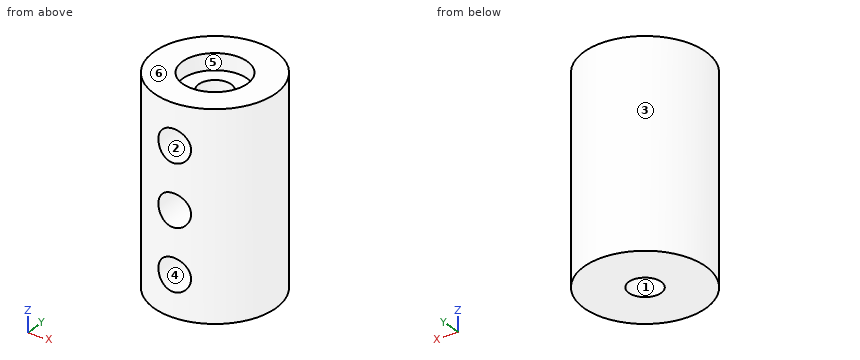
from build123d import *

# Parameters (mm, degrees)
F0_R     = 7.5
F0_R_2   = 2
F1_DEPTH = 12.5
F2_R     = 2
F3_DEPTH = 25
F4_R     = 4
F5_DEPTH = 2


with BuildPart() as f1:
    # F0 (on Top) → F1 (new body, symmetric)
    with BuildSketch(Plane.XY):
        Circle(F0_R)
        Circle(F0_R_2, mode=Mode.SUBTRACT)
    extrude(amount=F1_DEPTH, both=True)

    # F2 (on Front) → F3 (cut)
    with BuildSketch(Plane.XZ):
        with Locations((0, 7.5)):
            Circle(F2_R)
        with Locations((0, -7.5)):
            Circle(F2_R)
        Circle(F2_R)
    extrude(amount=F3_DEPTH, mode=Mode.SUBTRACT)

    # F4 (on face) → F5 (cut)
    with BuildSketch(Plane.XY.offset(12.5)):
        Circle(F4_R)
    extrude(amount=-F5_DEPTH, mode=Mode.SUBTRACT)


solid = f1.part
Geometry check sheet. Reference: the model listing, model coordinates, mm. Face numbers are marked on the shaded views. A direction names the side the tool comes from. Give positions to 0.01 mm unless a question says otherwise; leave off trailing zeros. Order: outer loops, then holes, each group sorted by start corner. A loop starts at its lowest first (then second) coordinate and runs counter-clockwise, first axis right, second up. Notation, with made-up numbers: (-9, -5.5) - (-5, -5.5) arc R6 cw to (-5, 4.5) - close; hole circle Ø11 at (-38.75, 38.5). An arc over 180 degrees is marked (long way). Answer as a JSON object with one key per item and string values.
(1) Cross-section at A-A (x = 0). Record the cut outline in (y, z).
Report:
{"outline": "(-7.5, -12.5) - (-2, -12.5) - (-2, -9.5) - (-7.5, -9.5) - close; (-7.5, -5.5) - (-2, -5.5) - (-2, -2) - (-7.5, -2) - close; (-7.5, 2) - (-2, 2) - (-2, 5.5) - (-7.5, 5.5) - close; (-7.5, 9.5) - (-2, 9.5) - (-2, 10.5) - (-4, 10.5) - (-4, 12.5) - (-7.5, 12.5) - close; (2, -12.5) - (7.5, -12.5) - (7.5, 12.5) - (4, 12.5) - (4, 10.5) - (2, 10.5) - close"}
(2) Cross-section at B-B (y = -4.5). Record the cut outline in (x, z).
Report:
{"outline": "(-6, -12.5) - (6, -12.5) - (6, 12.5) - (-6, 12.5) - close; hole circle Ø4 at (0, -7.5); hole circle Ø4 at (0, 0); hole circle Ø4 at (0, 7.5)"}
(3) Tool access check on the marked faces 4, 5 and 6. Record the directions out of +Z, -Z, +X, -X, +Y, -Y that give a thin tool (end or side, any length) a straight path to the whole face; none if there is none.
Report:
{"face 4": "-Y", "face 5": "+Z", "face 6": "+Z, +X, -X, +Y, -Y"}
(4) Material ranges on line 1 (Z direction, x = 0, y = -4.25); line 2 (Z direction, x = 0, y = -3); line 3 (X direction, y = -6, z = 0), recorded low to high.
Report:
{"line 1": "-12.5 to -9.5, -5.5 to -2, 2 to 5.5, 9.5 to 12.5", "line 2": "-12.5 to -9.5, -5.5 to -2, 2 to 5.5, 9.5 to 10.5", "line 3": "-4.5 to -2, 2 to 4.5"}
(5) Draft check along Y on the marked faces 1, 2 and 3. Enter one of: released by +Y, released by -Y, zero draft, split by the parting line, or undercut.
Report:
{"face 1": "undercut", "face 2": "zero draft", "face 3": "split by the parting line"}
(6) Cross-section at D-D (z = 5). Record the cut outline in (x, y).
Report:
{"outline": "circle Ø15 at (0, 0); hole circle Ø4 at (0, 0)"}
(7) Cross-section at C-C (y = -0.5). Record the cut outline in (x, z), then the cut area to 3 significant figures.
Report:
{"outline": "(-7.48, -12.5) - (-1.94, -12.5) - (-1.94, -8) arc R2 cw to (-1.94, -7) - (-1.94, -0.5) arc R2 cw to (-1.94, 0.5) - (-1.94, 7) arc R2 cw to (-1.94, 8) - (-1.94, 10.5) - (-3.97, 10.5) - (-3.97, 12.5) - (-7.48, 12.5) - close; (1.94, -12.5) - (7.48, -12.5) - (7.48, 12.5) - (3.97, 12.5) - (3.97, 10.5) - (1.94, 10.5) - (1.94, 8) arc R2 cw to (1.94, 7) - (1.94, 0.5) arc R2 cw to (1.94, -0.5) - (1.94, -7) arc R2 cw to (1.94, -8) - close", "area": "269 mm^2"}
(8) Depth check by flat-ended pin: pin 1 Ø3 at (x, z) = (4, -10) entering from +Y; pin 2 Ø3 at (y, z) = (4, -6) entering from +X. Enter the tip coordinate at first touch or a pass-through.
Report:
{"pin 1": "y = 7.07", "pin 2": "x = 7.07"}
